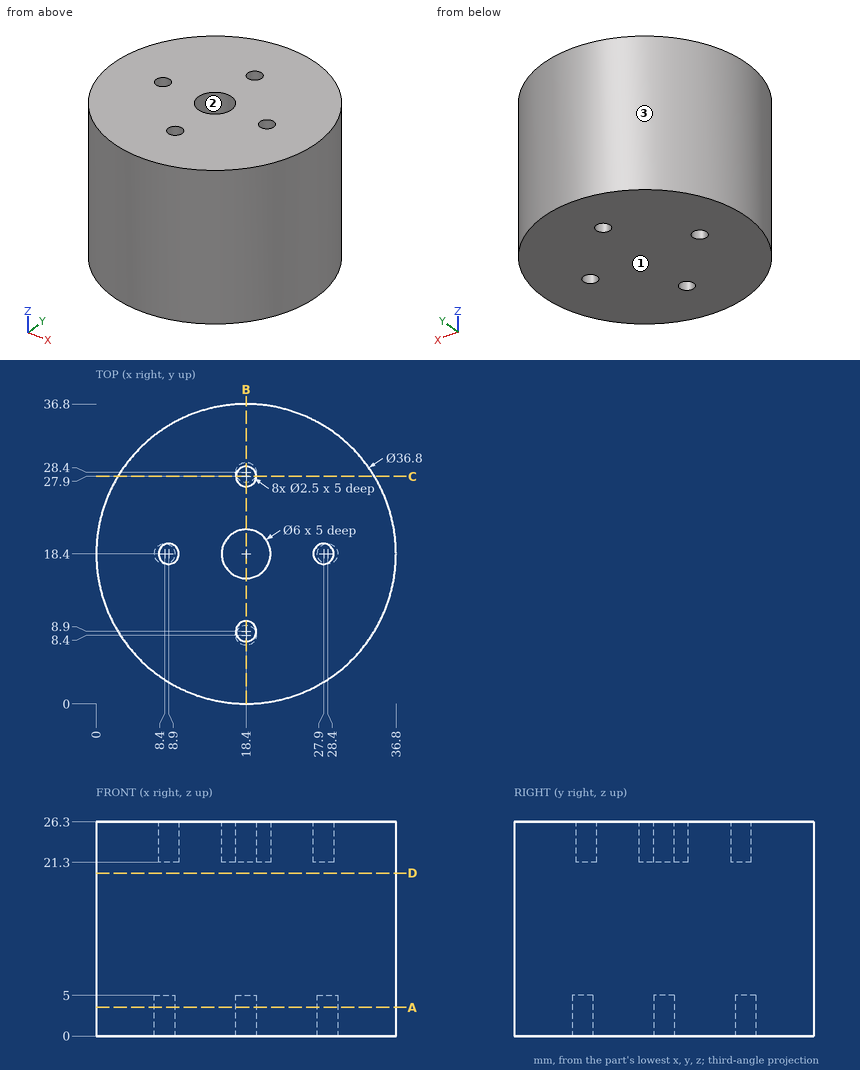
Design review of the part shown in the three views and the two pictorial views. Dimensions are in mm from the part's minimum x, y and z. Round coordinates to 2 decimals unless told otherwise and drop trailing zeros. Write each loop counter-clockwise with the first axis right and the second up, starting at its lowest first coordinate (ties: lowest second). Pieces come first, ordered by that corner, then holes. Notation, with made-up numbers: (-38, -13) -> (-14, -13) arc R32 ccw to (-14, 26) -> close; hole circle Ø10 at (66, 64). An arc over 180 degrees is marked (long way). Write item = value, one per line. Start each with the question number.
1) Take a section at A-A, the plane z = 3.5. State the section outline as (x, y) points.
2) Take a section at C-C, the plane y = 27.9. State the section outline as (x, z) points, plus the area to 3 significant figures.
3) Mouldability with a two-part tool opening along X and no side actions: class the marked faces 1, 2 and 3 as +X half, -X half, draft (parallel to the pull), parting line (faces both ways), or undercut.
4) Wall thickness on probe 1 along Y at (x, z) = (18.4, 23.75); probe 2 along Y at (x, z) = (18.4, 3.4); probe 3 along X at (y, z) = (20, 22.5): over which ranges is each line inside the solid? List them lowest first. Write a range as from..to.
5) Take a section at D-D, the plane z = 20. State the section outline as (x, y) points, plus the area to 3 significant figures.
6) Clearance check with flat-ended pins moving along their axes: pin 1 (1 mm diameter, centred on x = 23.5, z = 22, fed in from -Y); pin 2 (5 mm diameter, centred on y = 14.5, z = 17, fed in from -X); pin 3 (1.5 mm diameter, centred on y = 10, z = 5.5, fed in from +X). State where each tip first meets the part, or that it passes through.
7) Take a section at B-B, the plane x = 18.4. State the section outline as (y, z) points.
Results list:
q1.outline = circle Ø36.8 at (18.4, 18.4); hole circle Ø2.5 at (8.4, 18.4); hole circle Ø2.5 at (18.4, 8.4); hole circle Ø2.5 at (18.4, 28.4); hole circle Ø2.5 at (28.4, 18.4)
q2.outline = (2.64, 0) -> (17.25, 0) -> (17.25, 5) -> (19.55, 5) -> (19.55, 0) -> (34.16, 0) -> (34.16, 26.3) -> (19.65, 26.3) -> (19.65, 21.3) -> (17.15, 21.3) -> (17.15, 26.3) -> (2.64, 26.3) -> close
q2.area = 805 mm²
q3.face_1 = draft
q3.face_2 = undercut
q3.face_3 = parting line
q4.probe_1 = 0..7.65, 10.15..15.4, 21.4..26.65, 29.15..36.8
q4.probe_2 = 0..7.15, 9.65..27.15, 29.65..36.8
q4.probe_3 = 0.07..15.86, 20.94..36.73
q5.outline = circle Ø36.8 at (18.4, 18.4)
q5.area = 1,060 mm²
q6.pin_1 = 0.58
q6.pin_2 = 0.05
q6.pin_3 = 35.13
q7.outline = (0, 0) -> (7.15, 0) -> (7.15, 5) -> (9.65, 5) -> (9.65, 0) -> (27.15, 0) -> (27.15, 5) -> (29.65, 5) -> (29.65, 0) -> (36.8, 0) -> (36.8, 26.3) -> (29.15, 26.3) -> (29.15, 21.3) -> (26.65, 21.3) -> (26.65, 26.3) -> (21.4, 26.3) -> (21.4, 21.3) -> (15.4, 21.3) -> (15.4, 26.3) -> (10.15, 26.3) -> (10.15, 21.3) -> (7.65, 21.3) -> (7.65, 26.3) -> (0, 26.3) -> close
